Part model, mm, in its own coordinate system. Face numbers are marked on the shaded views. Give positions to 0.01 mm unless a question says otherwise; leave off trailing zeros. Loops run counter-clockwise (first coordinate to the right, second up) from the corner with the lowest first, then second, coordinate; pieces in that order, holes last. Notation, with made-up numbers: (-15, 68.25) -> (10, 68.25) arc R22 ccw to (10, 83.25) -> close; hole circle Ø10 at (8.25, -6). An arc over 180 degrees is marked (long way). One line per question, with ' | ' between items.
```python
from build123d import *

# Parameters (mm, degrees)
SKETCH_1_W          = 61.55
SKETCH_1_H          = 104.65
EXTRUDE_1_DEPTH     = 4.1
EXTRUDE_2_DEPTH     = 0.1
SKETCH_13_W         = 5
SKETCH_13_H         = 89
SKETCH_13_H_2       = 44
SKETCH_13_H_3       = 35
EXTRUDE_3_DEPTH     = 0.15
SWEEP_START         = -14.325
SWEEP_1_DEPTH       = 20
SWEEP_START_2       = -6.005
SWEEP_2_DEPTH       = 12
CUT_EXTRUDE_1_REACH = 65.813
SKETCH_21_W         = 3.5
SKETCH_21_H         = 10
SKETCH_22_W         = 5
SKETCH_22_H         = 5
EXTRUDE_4_DEPTH     = 1
SKETCH_22_3_W       = 0.5
SKETCH_22_3_H       = 1
EXTRUDE_5_DEPTH     = 0.5


# Read off the part's stored shape, not the designer's step: 扫描1, 扫描2
with BuildPart() as part:
    # 草图1 → 凸台-拉伸1 (new body)
    with BuildSketch(Plane.XY):
        Rectangle(SKETCH_1_W, SKETCH_1_H)
    extrude(amount=EXTRUDE_1_DEPTH)

    # 草图12 → 凸台-拉伸2 (add)
    with BuildSketch(Plane(origin=(0, 0, 0), x_dir=(-1, 0, 0), z_dir=(0, 0, -1))):
        with BuildLine():
            Line((-30.775, 5.675), (7.43097714, 5.675))
            ThreePointArc((7.43097714, 5.675), (8.96553195, 5.039366586), (9.601165364, 3.504811776))
            Line((9.601165364, 3.504811776), (9.601165364, -37.354811776))
            ThreePointArc((9.601165364, -37.354811776), (10.236798778, -38.889366586), (11.771353588, -39.525))
            Line((11.771353588, -39.525), (25.622658883, -39.525))
            ThreePointArc((25.622658883, -39.525), (27.157213692, -40.160633414), (27.792847106, -41.695188224))
            Line((27.792847106, -41.695188224), (27.792847106, -52.325))
            Line((27.792847106, -52.325), (-18.797778056, -52.325))
            Line((-18.797778056, -52.325), (-18.797778056, -16.495188224))
            ThreePointArc((-18.797778056, -16.495188224), (-19.43341147, -14.960633414), (-20.96796628, -14.325))
            Line((-20.96796628, -14.325), (-30.775, -14.325))
            Line((-30.775, -14.325), (-30.775, 5.675))
        make_face()
    extrude(amount=EXTRUDE_2_DEPTH)

    # 草图13 → 凸台-拉伸3 (add)
    with BuildSketch(Plane(origin=(0, 0, 0), x_dir=(-1, 0, 0), z_dir=(0, 0, -1))):
        with Locations((28.275, 7.825)):
            Rectangle(SKETCH_13_W, SKETCH_13_H)
        with Locations((-28.275, 30.325)):
            Rectangle(SKETCH_13_W, SKETCH_13_H_2)
        with Locations((-28.275, -34.825)):
            Rectangle(SKETCH_13_W, SKETCH_13_H_3)
    extrude(amount=EXTRUDE_3_DEPTH)

    # 扫描1 outline → 扫描1 (add)
    with BuildSketch(Plane(origin=(0, 0, 0), x_dir=(1, 0, 0), z_dir=(0, 1, 0)).offset(SWEEP_START)):
        with BuildLine():
            Line((30.775, 0), (33.688057754, 0))
            add(Edge.make_bspline(
                [(33.688057754, 0), (33.740094349, 0.030384855), (33.842167666, 0.089986814), (33.957599344, 0.199336205), (34.055275833, 0.337544191), (34.127351146, 0.503103592), (34.185512523, 0.716829871), (34.22259154, 0.985198024), (34.217211516, 1.305147843), (34.157564693, 1.596323551), (34.059081534, 1.841158616), (33.942865451, 2.037727084), (33.787885639, 2.222839862), (33.590692863, 2.391010577), (33.262024043, 2.589254607), (32.734303663, 2.759632394), (32.006537514, 2.830109489), (31.159482774, 2.834077419), (30.301363299, 2.787487983), (29.724318905, 2.754110628), (29.465689882, 2.739151029)],
                knots=[0, 0, 0, 0, 0.022394077, 0.043927504, 0.06594757, 0.090294372, 0.118608139, 0.159927725, 0.205818656, 0.25470695, 0.285347598, 0.317202924, 0.350795774, 0.386909923, 0.42653968, 0.513682935, 0.622352859, 0.744271405, 0.885383452, 1, 1, 1, 1], degree=3))
            Line((29.465689882, 2.739151029), (16.573878781, 2.449987427))
            Line((16.573878781, 2.449987427), (16.576121219, 2.350012573))
            Line((16.576121219, 2.350012573), (29.468846669, 2.639196684))
            add(Edge.make_bspline(
                [(33.66280425, 0.1), (33.701165427, 0.12284106), (33.77641348, 0.167645351), (33.88316176, 0.26642733), (33.966512799, 0.385635161), (34.032372412, 0.535121016), (34.087077442, 0.736116999), (34.122405453, 0.991235451), (34.117202793, 1.294498152), (34.060993674, 1.568287463), (33.969014807, 1.796825073), (33.860895162, 1.979670143), (33.716718378, 2.151914558), (33.532385119, 2.309217599), (33.222301128, 2.496419386), (32.71697835, 2.660403065), (32.002919105, 2.730108386), (31.162255161, 2.734053994), (30.308880523, 2.687749647), (29.728825185, 2.654223135), (29.468846669, 2.639196684)],
                knots=[0, 0, 0, 0, 0.022394077, 0.043927504, 0.06594757, 0.090294372, 0.118608139, 0.159927725, 0.205818656, 0.25470695, 0.285347598, 0.317202924, 0.350795774, 0.386909923, 0.42653968, 0.513682935, 0.622352859, 0.744271405, 0.885383452, 1, 1, 1, 1], degree=3))
            Line((33.66280425, 0.1), (30.775, 0.1))
            Line((30.775, 0.1), (30.775, 0))
        make_face()
    extrude(amount=SWEEP_1_DEPTH)

    # 扫描2 outline → 扫描2 (add)
    with BuildSketch(Plane.YZ.offset(SWEEP_START_2)):
        with BuildLine():
            add(Edge.make_bspline(
                [(-52.325, 3), (-52.460602146, 2.893750812), (-52.722932906, 2.688205168), (-53.009596176, 2.286811717), (-53.236110287, 1.775702365), (-53.359405567, 1.129360272), (-53.359062945, 0.238903879), (-53.229025848, -0.783276027), (-52.933769169, -1.695551183), (-52.526896187, -2.296702581), (-52.132903591, -2.646463291), (-51.661381942, -2.902920315), (-50.942443081, -3.139445785), (-49.94695976, -3.245581242), (-48.75217865, -3.148841506), (-47.635336399, -2.915993871), (-46.974786487, -2.629681533), (-46.67140425, -2.498181891)],
                knots=[0, 0, 0, 0, 0.043360734, 0.083884028, 0.123581472, 0.184240498, 0.247655218, 0.345647149, 0.439787351, 0.484257058, 0.527954224, 0.57258299, 0.619125258, 0.717850297, 0.820060491, 0.917356055, 1, 1, 1, 1], degree=3))
            Line((-52.325, 3), (-52.325, 3.1))
            add(Edge.make_bspline(
                [(-52.325, 3.1), (-52.468608186, 2.993246309), (-52.746427128, 2.786724673), (-53.057421939, 2.375880968), (-53.306118632, 1.849117463), (-53.443742145, 1.185180174), (-53.453016098, 0.27667256), (-53.326868431, -0.756873175), (-53.036730374, -1.692169497), (-52.625569397, -2.326691599), (-52.219376389, -2.703311261), (-51.732982096, -2.977735995), (-50.993631594, -3.23110648), (-49.979600344, -3.345075131), (-48.766358256, -3.253086402), (-47.634912854, -3.022591855), (-46.957432057, -2.73424992), (-46.646273679, -2.601818109)],
                knots=[0, 0, 0, 0, 0.043360734, 0.083884028, 0.123581472, 0.184240498, 0.247655218, 0.345647149, 0.439787351, 0.484257058, 0.527954224, 0.57258299, 0.619125258, 0.717850297, 0.820060491, 0.917356055, 1, 1, 1, 1], degree=3))
            Line((-46.646273679, -2.601818109), (-28.485, -2.601818109))
            Line((-28.485, -2.601818109), (-28.485, -2.498181891))
            Line((-28.485, -2.498181891), (-46.67140425, -2.498181891))
        make_face()
    extrude(amount=SWEEP_2_DEPTH)

    # 草图21 → 切除-拉伸1 (cut, up to next)
    with BuildSketch(Plane(origin=(0, 0, -2.601818109), x_dir=(-1, 0, 0), z_dir=(0, 0, -1)), mode=Mode.PRIVATE) as cut_extrude_1_sk1:
        with Locations((-4.245, -33.485)):
            Rectangle(SKETCH_21_W, SKETCH_21_H)
    cut_extrude_1_tool1 = extrude(cut_extrude_1_sk1.sketch, amount=-CUT_EXTRUDE_1_REACH, mode=Mode.PRIVATE) & part.part
    # 草图21 → 切除-拉伸1 (cut, up to next)
    with BuildSketch(Plane(origin=(0, 0, -2.601818109), x_dir=(-1, 0, 0), z_dir=(0, 0, -1)), mode=Mode.PRIVATE) as cut_extrude_1_sk2:
        with Locations((4.255, -33.485)):
            Rectangle(SKETCH_21_W, SKETCH_21_H)
    cut_extrude_1_tool2 = extrude(cut_extrude_1_sk2.sketch, amount=-CUT_EXTRUDE_1_REACH, mode=Mode.PRIVATE) & part.part
    add(cut_extrude_1_tool1.solids().sort_by_distance((4.245, -33.485, -2.601818))[0], mode=Mode.SUBTRACT)
    add(cut_extrude_1_tool2.solids().sort_by_distance((-4.255, -33.485, -2.601818))[0], mode=Mode.SUBTRACT)

    # 草图22 → 凸台-拉伸4 (add)
    with BuildSketch(Plane(origin=(0, 0, -2.601818109), x_dir=(-1, 0, 0), z_dir=(0, 0, -1))):
        with Locations((0.005, -43.046273679)):
            Rectangle(SKETCH_22_W, SKETCH_22_H)
    extrude(amount=EXTRUDE_4_DEPTH)

    # 草图22<3> → 凸台-拉伸5 (add)
    with BuildSketch(Plane(origin=(0, 0, -2.601818109), x_dir=(-1, 0, 0), z_dir=(0, 0, -1))):
        with Locations((-3.445, -39.485)):
            Rectangle(SKETCH_22_3_W, SKETCH_22_3_H)
        with Locations((-2.445, -39.485)):
            Rectangle(SKETCH_22_3_W, SKETCH_22_3_H)
        with Locations((-1.445, -39.485)):
            Rectangle(SKETCH_22_3_W, SKETCH_22_3_H)
        with Locations((-0.445, -39.485)):
            Rectangle(SKETCH_22_3_W, SKETCH_22_3_H)
        with Locations((0.555, -39.485)):
            Rectangle(SKETCH_22_3_W, SKETCH_22_3_H)
        with Locations((1.555, -39.485)):
            Rectangle(SKETCH_22_3_W, SKETCH_22_3_H)
        with Locations((2.555, -39.485)):
            Rectangle(SKETCH_22_3_W, SKETCH_22_3_H)
        with Locations((3.555, -39.485)):
            Rectangle(SKETCH_22_3_W, SKETCH_22_3_H)
    extrude(amount=EXTRUDE_5_DEPTH)


solid = part.part
```
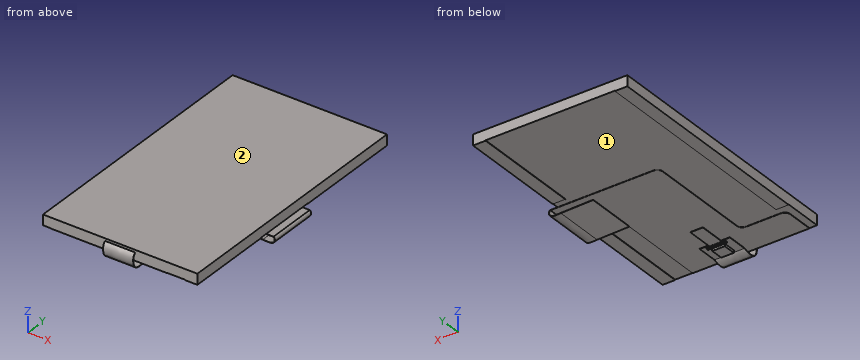
1) Saw through at B-B (x = 23). Give the cut face in (y, z) (3 decimals).
Found:
outline: (-52.325, 0) -> (-14.325, 0) -> (-14.325, -0.1) -> (5.675, -0.1) -> (5.675, 0) -> (52.325, 0) -> (52.325, 4.1) -> (-52.325, 4.1) -> close; (-14.325, -2.594) -> (5.675, -2.594) -> (5.675, -2.494) -> (-14.325, -2.494) -> close
2) Pull direction X, two halves, no side cores. Call the marked faces 1 and 2: pulls with the +X half, pulls with the -X half, needs draft (parallel to the pull), parting line crosses it, or undercut.
Found:
face 1: undercut | face 2: needs draft
3) Saw through at C-C (x = 7.5). Give the cut face in (y, z) (3 decimals).
Found:
outline: (-52.325, -0.1) -> (5.675, -0.1) -> (5.675, 0) -> (52.325, 0) -> (52.325, 4.1) -> (-52.325, 4.1) -> close
4) Drill centre lines: line 1 (Z direction, x = -12, y = 22); line 2 (Z direction, x = 11, y = -31.5); line 3 (X direction, y = 22.5, z = 1) (3 decimals). Where is each one in solid material? Low to high.
Found:
line 1: 0 to 4.1 | line 2: -0.1 to 4.1 | line 3: -30.775 to 30.775
5) Pin check, flat tips, straight feed: P1, Ø6, axis at x = 26, y = -28, coming from the -Z side; P2, Ø0.6, axis at y = -39.5, z = -3, coming from the -X side (3 decimals); P3, Ø1, axis at y = 16, z = 0.5, coming from the +X side (3 decimals). Stop position of each tip, or through.
Found:
P1: z = -0.15 | P2: x = -3.805 | P3: x = 30.775
6) Saw through at D-D (x = -18). Give the cut face in (y, z) (3 decimals), and give its area (3 significant figures).
Found:
outline: (-52.325, -0.1) -> (-39.525, -0.1) -> (-39.525, 0) -> (52.325, 0) -> (52.325, 4.1) -> (-52.325, 4.1) -> close | area: 430 mm2
7) Saw through at A-A (y = 37). Give the cut face in (x, z) (3 decimals), and give its area (3 significant figures).
Found:
outline: (-30.775, -0.15) -> (-25.775, -0.15) -> (-25.775, 0) -> (25.775, 0) -> (25.775, -0.15) -> (30.775, -0.15) -> (30.775, 4.1) -> (-30.775, 4.1) -> close | area: 254 mm2
